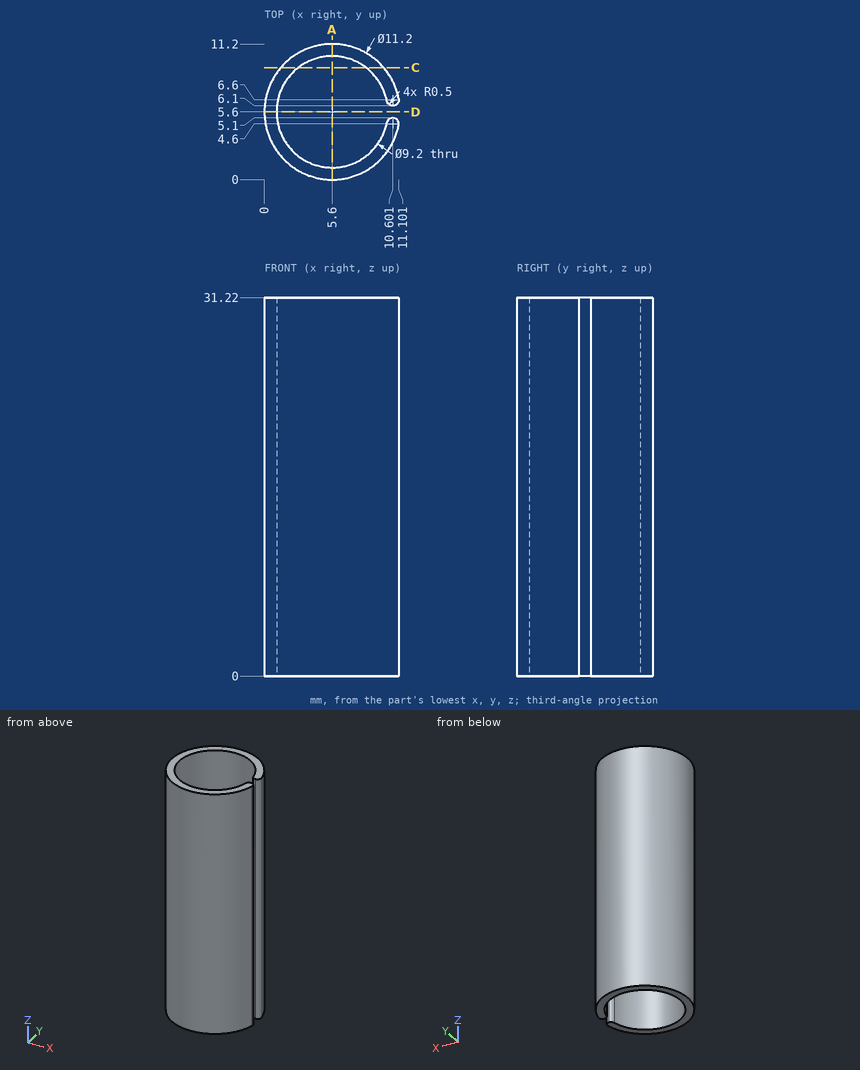
Geometry check sheet. Reference: drawing and pictorial views, mm from the part's lowest x, y, z. Coordinates: 2 decimals unless noted, no trailing zeros. Write each loop counter-clockwise with the first axis right and the second up, starting at its lowest first coordinate (ties: lowest second). Pieces come first, ordered by that corner, then holes.
Item 1: Cross-section at A-A on x = 5.6. Record the boundary of the cut face in (y, z).
Numbers:
outline: (0, 0) - (1, 0) - (1, 31.22) - (0, 31.22) - close; (10.2, 0) - (11.2, 0) - (11.2, 31.22) - (10.2, 31.22) - close
Item 2: Cross-section at C-C on y = 9.25. Record the boundary of the cut face in (x, z), then the cut area to 3 significant figures.
Numbers:
outline: (1.35, 0) - (2.8, 0) - (2.8, 31.22) - (1.35, 31.22) - close; (8.4, 0) - (9.85, 0) - (9.85, 31.22) - (8.4, 31.22) - close
area: 90.4 mm2
Item 3: Scan lines: probe 1 along Y at (x, z) = (5.6, 10); probe 2 along Y at (x, z) = (7.25, 22); probe 3 along X at (y, z) = (9.25, 15). Record each from-to range of solid material in increasing order.
Numbers:
probe 1: y = 0 to 1, 10.2 to 11.2
probe 2: y = 0.25 to 1.31, 9.89 to 10.95
probe 3: x = 1.35 to 2.8, 8.4 to 9.85
Item 4: Cross-section at D-D on y = 5.6. Record the boundary of the cut face in (x, z).
Numbers:
outline: (0, 0) - (1, 0) - (1, 31.22) - (0, 31.22) - close
Item 5: Depth check by flat-ended pin: pin 1 Ø3 at (x, z) = (3, 11.5) entering from +Y; pin 2 Ø3 at (x, z) = (2.5, 11) entering from +Y; pin 3 Ø3 at (y, z) = (4.5, 5) entering from +X; pin 4 Ø2 at (x, z) = (8.5, 10) entering from -Y. Enter the tip coordinate at first touch or a pass-through.
Numbers:
pin 1: stops at y = 11.09
pin 2: stops at y = 10.97
pin 3: stops at x = 11.1
pin 4: stops at y = 0.33
